Source: CAD feature listing. Evaluate the final solid. Frame: model axes, mm. Face numbers are marked on the shaded views. Coordinates: 2 decimals unless noted, no trailing zeros. Write each loop counter-clockwise with the first axis right and the second up, starting at its lowest first coordinate (ties: lowest second). Pieces come first, ordered by that corner, then holes. Notation, with made-up numbers: (11.5, 85.5) - (48.5, 85.5) arc R29 ccw to (48.5, 118.5) - close; hole circle Ø6 at (85, 41.5). An arc over 180 degrees is marked (long way). One line per question, with ' | ' between items.
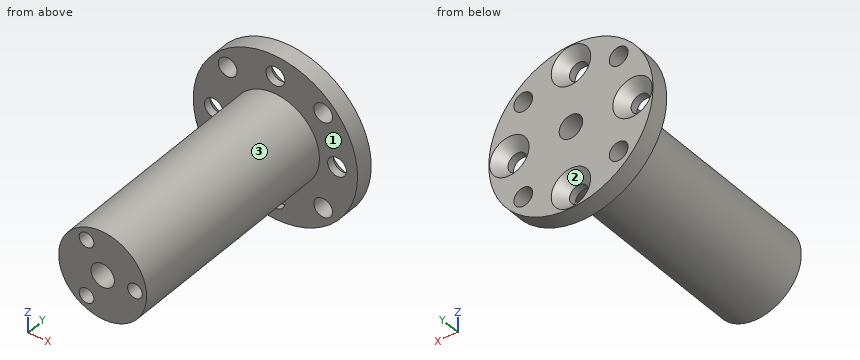
from build123d import *

# Parameters (mm, degrees)
F_4_0_4_DURCHMESSER_BOHRUNG1_D       = 4
F_4_0_4_DURCHMESSER_BOHRUNG1_DEPTH   = 41
KREISMUSTER1_COUNT                   = 3
KREISMUSTER2_COUNT                   = 4
F_3_2_3_2_DURCHMESSER_BOHRUNG1_D     = 3.2
F_3_2_3_2_DURCHMESSER_BOHRUNG1_DEPTH = 3.001
KREISMUSTER3_COUNT                   = 4


with BuildPart() as part:
    # Skizze1 → Rotation1 (revolve)
    with BuildSketch(Plane.XY):
        Polygon((0, 0), (14, 0), (14, -3), (7.5, -3), (7.5, -41), (0, -41), align=None)
    revolve(axis=Axis((0, 9.414893617, 0), (0, -1, 0)))

    # Ø4.0 (4) Durchmesser Bohrung1
    with Locations(Plane(origin=(0, 0, 0), x_dir=(1, 0, 0), z_dir=(0, 1, 0))):
        with Locations((0, 0)):
            Hole(F_4_0_4_DURCHMESSER_BOHRUNG1_D / 2, depth=F_4_0_4_DURCHMESSER_BOHRUNG1_DEPTH)

    # Skizze4 → M3 Gewindebohrung1 (revolve, cut)
    with BuildSketch(Plane(origin=(5.5, -41, 0), x_dir=(0, 0, -1), z_dir=(1, 0, 0))):
        Polygon((0, 0), (0, 12.751075774), (1.25, 12), (1.25, 0), align=None)
    m3_gewindebohrung1 = revolve(axis=Axis((5.5, -47.35, 0), (0, 1, 0)), mode=Mode.SUBTRACT)

    # Kreismuster1: M3 Gewindebohrung1 ×3 about axis
    kreismuster1_axis = Axis((0, 0, 0), (0, 1, 0))
    for i in range(1, KREISMUSTER1_COUNT):
        add(m3_gewindebohrung1.rotate(kreismuster1_axis, i * 360 / KREISMUSTER1_COUNT), mode=Mode.SUBTRACT)

    # Skizze6 → Formsenkung für M3 Senkschraube mit Innensechskant1 (revolve, cut)
    with BuildSketch(Plane(origin=(0, 0, -10.5), x_dir=(0, 0, 1), z_dir=(1, 0, 0))):
        Polygon((0, 0), (0, 3.001), (1.6, 3.001), (1.6, 1.76), (3.36, 0), align=None)
    formsenkung_f_r_m3_senkschraube_mit_inne = revolve(axis=Axis((0, 6.35, -10.5), (0, -1, 0)), mode=Mode.SUBTRACT)

    # Kreismuster2: Formsenkung für M3 Senkschraube mit Innensechskant1 ×4 about axis
    kreismuster2_axis = Axis((0, 0, 0), (0, 1, 0))
    for i in range(1, KREISMUSTER2_COUNT):
        add(formsenkung_f_r_m3_senkschraube_mit_inne.rotate(kreismuster2_axis, i * 360 / KREISMUSTER2_COUNT), mode=Mode.SUBTRACT)

    # Ø3.2 (3.2) Durchmesser Bohrung1
    with Locations(Plane(origin=(0, 0, 0), x_dir=(1, 0, 0), z_dir=(0, 1, 0))):
        with Locations((-8.131727984, 8.131727984)):
            f_3_2_3_2_durchmesser_bohrung1 = Hole(F_3_2_3_2_DURCHMESSER_BOHRUNG1_D / 2, depth=F_3_2_3_2_DURCHMESSER_BOHRUNG1_DEPTH)

    # Kreismuster3: Ø3.2 (3.2) Durchmesser Bohrung1 ×4 about axis
    kreismuster3_axis = Axis((0, 0, 0), (0, 1, 0))
    for i in range(1, KREISMUSTER3_COUNT):
        add(f_3_2_3_2_durchmesser_bohrung1.rotate(kreismuster3_axis, i * 360 / KREISMUSTER3_COUNT), mode=Mode.SUBTRACT)


solid = part.part
Item 1: Ray query, line 1 along Z through (x, y) = (0, -15.5); line 2 along Z through (x, y) = (-7, -1.5); line 3 along Z through (x, y) = (10.5, -2.05). Return the intervals inside material, ascending. Write a range as [from, to].
Check sheet entries:
line 1: [-7.5, -2], [2, 7.5] | line 2: [-12.12, -9.26], [-7, 7], [9.26, 12.12] | line 3: [-9.26, -1.6], [1.6, 9.26]
Item 2: Cut plane A-A on x = 0. Return loops of the section in (y, z).
Check sheet entries:
outline: (-41, -7.5) - (-3, -7.5) - (-3, -8.9) - (-1.76, -8.9) - (0, -7.14) - (0, -2) - (-41, -2) - close; (-41, 2) - (0, 2) - (0, 7.14) - (-1.76, 8.9) - (-3, 8.9) - (-3, 7.5) - (-41, 7.5) - close; (-3, -14) - (0, -14) - (0, -13.86) - (-1.76, -12.1) - (-3, -12.1) - close; (-3, 12.1) - (-1.76, 12.1) - (0, 13.86) - (0, 14) - (-3, 14) - close
Item 3: Cut plane C-C on z = 10.5. Return loops of the section in (x, y), and give its area (3 significant figures).
Check sheet entries:
outline: (-9.26, -3) - (-1.6, -3) - (-1.6, -1.76) - (-3.36, 0) - (-9.26, 0) - close; (1.6, -3) - (9.26, -3) - (9.26, 0) - (3.36, 0) - (1.6, -1.76) - close | area: 42.9 mm²
Item 4: Cut plane D-D on x = -10.5. Return loops of the section in (y, z).
Check sheet entries:
outline: (-3, -9.26) - (0, -9.26) - (0, -3.36) - (-1.76, -1.6) - (-3, -1.6) - close; (-3, 1.6) - (-1.76, 1.6) - (0, 3.36) - (0, 9.26) - (-3, 9.26) - close
Item 5: Cut plane B-B on y = -22. Return loops of the section in (x, z), and give its area (3 significant figures).
Check sheet entries:
outline: circle Ø15 at (0, 0); hole circle Ø4 at (0, 0) | area: 164 mm²
Item 6: Pin query (flat end, axial travel): pin 1 Ø8 at (x, y) = (4, -7.5) entering from +Z; pin 2 Ø12 at (x, y) = (-7, -33.5) entering from -Z; pin 3 Ø4 at (x, z) = (0, -10.5) entering from -Y. Return the tip coordinate at first contact, or that it passes through.
Check sheet entries:
pin 1: z = 7.5 | pin 2: z = -7.43 | pin 3: y = -3
Item 7: Mould query, pull axis Z, two halves, no side actions, for the marked faces 1, 2 and 3. Classes: pulls with the +Z half, pulls with the -Z half, needs draft (parallel to the pull), parting line crosses it, or undercut.
Check sheet entries:
face 1: needs draft | face 2: undercut | face 3: parting line crosses it
